Read the model definition and answer for the solid it produces. Units are mm, in the model's axes. A direction names the side the tool comes from. Coordinates: 2 decimals unless noted, no trailing zeros. Loops run counter-clockwise (first coordinate to the right, second up) from the corner with the lowest first, then second, coordinate; pieces in that order, holes last. Notation, with made-up numbers: (52, -10.75) - (109, -10.75) arc R9 cw to (109, -1.75) - close; hole circle Ø5 at (-9.75, -11). An arc over 180 degrees is marked (long way). Use CSV: the item, a comma, the result in double quotes.
```python
from build123d import *

# Parameters (mm, degrees)
F1_DEPTH = 127


with BuildPart() as f1:
    # F0 (on Front) → F1 (new body)
    with BuildSketch(Plane.XZ):
        with BuildLine():
            Line((3, 60.958375), (3, 58.212375))
            ThreePointArc((3, 58.212375), (0, 55.212375), (-3, 58.212375))
            Line((-3, 58.212375), (-3.014112, 58.212375))
            Line((-3.014112, 58.212375), (-3.014112, 60.958375))
            Line((-3.014112, 60.958375), (-12.7, 60.958375))
            Line((-12.7, 60.958375), (-12.7, 48.258375))
            Line((-12.7, 48.258375), (12.7, 48.258375))
            Line((12.7, 48.258375), (12.7, 60.958375))
            Line((12.7, 60.958375), (3, 60.958375))
        make_face()
    extrude(amount=F1_DEPTH)


solid = f1.part
```
Q1. The part is cut by section B-B on x = 0. Determine the outline of the cut face in (y, z), and give its area (3 significant figures).
Reported:
outline,"(-127, 48.26) - (0, 48.26) - (0, 55.21) - (-127, 55.21) - close"
area,"883 mm²"
Q2. Find the intervals of material crossed by probe 1 along X at (y, z) = (-74.5, 57.5); probe 2 along X at (y, z) = (-83, 56.5); probe 3 along Z at (x, y) = (1.25, -47.5), in increasing order. Write a range as [from, to].
Reported:
probe 1,"x = [-12.7, -2.91], [2.91, 12.7]"
probe 2,"x = [-12.7, -2.46], [2.46, 12.7]"
probe 3,"z = [48.26, 55.49]"
Q3. For a pull along X with two mould halves and no side action, classify faces 3 (the face through (12.7, -63, 55)), 4 (the face through (-3.014, -63, 60)), 5 (the face through (-8, -63, 60.958)) as +X half, -X half, draft (parallel to the pull), parting line (faces both ways), or undercut.
Reported:
face 3,"+X half"
face 4,"undercut"
face 5,"draft"
Q4. Given P1, Ø3, axis at x = 2, y = -85, coming from the +Z side, flat-ended and moving along its own axis, determine where the tip first touches the part or whether it passes through.
Reported:
P1,"stops at z = 60.96"
Q5. A tool of negligible diameter and unlimited length cuts with its end or side. For faces 1 (the face through (3, -63, 60)), 2 (the face through (-12.7, -63, 55)), from which of +Z, -Z, +X, -X, +Y, -Y can it reach the whole face along a straight path? Write none if from no direction.
Reported:
face 1,"+Z, +Y, -Y"
face 2,"+Z, -Z, -X, +Y, -Y"
